from build123d import *

# Parameters (mm, degrees)
EXTRUDE_1_DEPTH          = 40
SKETCH_3_W               = 4
SKETCH_3_H               = 32
EXTRUDE_2_DEPTH          = 160
EXTRUDE_3_DEPTH          = 40
SKETCH_6_W               = 38
SKETCH_6_H               = 4
EXTRUDE_4_DEPTH          = 40
CUT_EXTRUDE_1_DEPTH      = 226.778652667
CUT_EXTRUDE_1_DEPTH_BACK = 226.778652667
SKETCH_4_W               = 10
SKETCH_4_H               = 10


with BuildPart() as part:
    # 草图2 → 凸台-拉伸1 (new body)
    with BuildSketch(Plane(origin=(0, 0, 0), x_dir=(1, 0, 0), z_dir=(0, 1, 0))):
        with BuildLine():
            Line((-40, -80), (40, -80))
            ThreePointArc((40, -80), (96.568542495, -56.568542495), (120, 0))
            Line((120, 0), (120, 16))
            Line((120, 16), (124, 16))
            Line((124, 16), (124, -16))
            Line((124, -16), (122.462112512, -16))
            ThreePointArc((122.462112512, -16), (93.441556864, -64.807406984), (40, -84))
            Line((40, -84), (-40, -84))
            ThreePointArc((-40, -84), (-93.441556864, -64.807406984), (-122.462112512, -16))
            Line((-122.462112512, -16), (-124, -16))
            Line((-124, -16), (-124, 16))
            Line((-124, 16), (-120, 16))
            Line((-120, 16), (-120, 0))
            ThreePointArc((-120, 0), (-96.568542495, -56.568542495), (-40, -80))
        make_face()
    extrude(amount=EXTRUDE_1_DEPTH)

    # 草图3 → 凸台-拉伸2 (add)
    with BuildSketch(Plane.XZ):
        with Locations((-122, 0)):
            Rectangle(SKETCH_3_W, SKETCH_3_H)
        with Locations((122, 0)):
            Rectangle(SKETCH_3_W, SKETCH_3_H)
    extrude(amount=EXTRUDE_2_DEPTH)

    # 草图5 → 凸台-拉伸3 (add)
    with BuildSketch(Plane(origin=(0, 40, 0), x_dir=(1, 0, 0), z_dir=(0, 1, 0))):
        Polygon((-40, -84), (-78, -84), (-78, -74.913283201), (-55.5334574, -80.946187921), (52.897278528, -80.946187921), (78, -72.607731722), (78, -84), (40, -84), align=None)
    extrude(amount=-EXTRUDE_3_DEPTH)

    # 草图6 → 凸台-拉伸4 (add)
    with BuildSketch(Plane(origin=(0, 40, 0), x_dir=(1, 0, 0), z_dir=(0, 1, 0))):
        with Locations((-59, -82)):
            Rectangle(SKETCH_6_W, SKETCH_6_H)
        with Locations((59, -82)):
            Rectangle(SKETCH_6_W, SKETCH_6_H)
    extrude(amount=EXTRUDE_4_DEPTH)

    # 草图4 → 切除-拉伸1 (cut, two sides: drawn at the far end of the back side and taken through both)
    with BuildSketch(Plane.XY.offset(84).offset(-CUT_EXTRUDE_1_DEPTH_BACK)):
        with Locations((0, 7.906009126)):
            Rectangle(SKETCH_4_W, SKETCH_4_H)
    extrude(amount=CUT_EXTRUDE_1_DEPTH + CUT_EXTRUDE_1_DEPTH_BACK, mode=Mode.SUBTRACT)


solid = part.part
Work out the finished part from the listing and answer in its coordinate system (mm). A direction names the side the tool comes from. Round coordinates to 2 decimals unless told otherwise and drop trailing zeros. Order: outer loops, then holes, each group sorted by start corner. A loop starts at its lowest first (then second) coordinate and runs counter-clockwise, first axis right, second up. Notation, with made-up numbers: M 2.5,69 L 35.5,69 A28 cw 35.5,88 Z; hole C 51,-34.75 d4. An arc over 180 degrees is marked long. One line per item, written item: value.
Q1. For faces 5 (the face through (78, 32, 80)), 6 (the face through (59, 60, 80)), 7 (the face through (120, -59, 0)), 8 (the face through (-97.19, 19.72, 55.94)), 9 (the face through (-1, 31, 84)), determine the directions among +Z, -Z, +X, -X, +Y, -Y from which every point of the face is accessible in a straight line to the end or side of a thin tool.
Derived:
face 5: +Z, +X, +Y, -Y
face 6: -Z, +X, -X, +Y
face 7: -Z, -Y
face 8: -Z, +Y, -Y
face 9: +Z, +X, -X, +Y, -Y
Q2. Flat-ended cylindrical pins translate along their axes: pin 1 (2 mm diameter, centred on x = 122, y = -72.5, fed in from +Z); pin 2 (4.5 mm diameter, centred on y = 51.5, z = 82, fed in from +X); pin 3 (3 mm diameter, centred on y = 10, z = 82.5, fed in from -X). Find the tip coordinate at first contact, or state that the pin passes through.
Derived:
pin 1: z = 16
pin 2: x = 78
pin 3: x = -78
Q3. Find section B-B on z = 46.5. Write down the section's boundary in (x, y).
Derived:
outline: M -109.96,0 L -105.1,0 L -105.1,40 L -109.96,40 Z; M 105.1,0 L 109.96,0 L 109.96,40 L 105.1,40 Z
Q4. Find section A-A on y = 10. Write down the section's boundary in (x, z), then the cut area to 3 significant figures.
Derived:
outline: M -124,-16 L -120,-16 L -120,0 A80 cw -40,80 L -5,80 L -5,84 L -78,84 L -78,74.91 A84 ccw -122.46,16 L -124,16 Z; M 5,80 L 40,80 A80 cw 120,0 L 120,-16 L 124,-16 L 124,16 L 122.46,16 A84 ccw 78,74.91 L 78,84 L 5,84 Z
area: 1,680 mm²
Q5. Find section C-C on y = 56. Write down the section's boundary in (x, z), then the cut area to 3 significant figures.
Derived:
outline: M -78,80 L -40,80 L -40,84 L -78,84 Z; M 40,80 L 78,80 L 78,84 L 40,84 Z
area: 304 mm²
Q6. Determine the mould class of faces 1 (the face through (-59, 60, 80)), 2 (the face through (95.94, 19.72, 57.19)), 3 (the face through (-78, 31, 81)), 4 (the face through (-1, 20, 80)) for opening direction X: released by +X, released by -X, zero draft, split by the parting line, or undercut.
Derived:
face 1: zero draft
face 2: undercut
face 3: released by -X
face 4: undercut
Q7. Find section D-D on x = -15. Write down the section's boundary in (y, z), then the cut area to 3 significant figures.
Derived:
outline: M 0,80 L 40,80 L 40,84 L 0,84 Z
area: 160 mm²
Q8. Straight lines are drawn through the part: line 1 (X direction, y = -113.5, z = -1.5); line 2 (Z direction, x = 38, y = 20.5); line 3 (X direction, y = 2, z = 43). For each, find the intervals that lie inside material, in ascending order.
Derived:
line 1: -124 to -120, 120 to 124
line 2: 80 to 84
line 3: -112.16 to -107.46, 107.46 to 112.16
